For this review, take the finished solid that the model builds, in its own axes (mm). A direction names the side the tool comes from. Round coordinates to 2 decimals unless told otherwise and drop trailing zeros. Order: outer loops, then holes, each group sorted by start corner. A loop starts at its lowest first (then second) coordinate and runs counter-clockwise, first axis right, second up. Notation, with made-up numbers: (30.25, -23.75) -> (54.25, -23.75) arc R27 ccw to (54.25, -3.75) -> close; hole circle Ø7 at (34.5, 21.5). An arc over 180 degrees is marked (long way). Answer in a Markdown table with one row per item.
```python
from build123d import *

# Parameters (mm, degrees)
PAD_DEPTH       = 40
POCKET_DEPTH    = 19
POCKET001_DEPTH = 19
FILLET_R        = 1
FILLET001_R     = 1.8


with BuildPart() as part:
    # Sketch → Pad (new body)
    with BuildSketch(Plane.XY):
        Polygon((0, 0), (0, -55), (5, -55), (45, -15), (45, 0), (41, 0), (41, -10), (5, -10), (5, 0), align=None)
    extrude(amount=PAD_DEPTH)

    # Sketch001 (on Face10 of Pad) → Pocket (cut)
    with BuildSketch(Plane(origin=(0, 0, 0), x_dir=(1, 0, 0), z_dir=(0, 0, -1))):
        Polygon((5, 12.5), (5, 50.5), (41, 12.5), align=None)
    extrude(amount=-POCKET_DEPTH, mode=Mode.SUBTRACT)

    # Sketch002 (on Face5 of Pocket) → Pocket001 (cut)
    with BuildSketch(Plane.XY.offset(40)):
        Polygon((5, -12.5), (41, -12.5), (5, -50.5), align=None)
    extrude(amount=-POCKET001_DEPTH, mode=Mode.SUBTRACT)

    # Fillet
    fillet_edges = [part.edges().sort_by_distance(p)[0] for p in [
        (5, 0, 20),
        (5, -10, 20),
        (45, -15, 20),
        (45, 0, 20),
        (41, 0, 20),
        (5, -55, 20),
        (41, -10, 20),
        (41, -12.5, 30.5),
        (5, -12.5, 30.5),
        (5, -50.5, 30.5),
        (5, -12.5, 9.5),
        (5, -50.5, 9.5),
        (41, -12.5, 9.5),
    ]]
    fillet(fillet_edges, radius=FILLET_R)

    # Fillet001
    fillet001_edges = [part.edges().sort_by_distance(p)[0] for p in [
        (23, -10, 40),
        (23, -10, 0),
    ]]
    fillet(fillet001_edges, radius=FILLET001_R)


solid = part.part
```
Q1. Clearance check with flat-ended pins moving along their axes: pin 1 Ø15 at (x, z) = (30.5, 31) entering from -Y; pin 2 Ø15 at (y, z) = (-34, 34) entering from +X; pin 3 Ø10.5 at (x, y) = (17, -26.5) entering from +Z. State where each tip first meets the part, or that it passes through.
Answer key:
| item | result |
|---|---|
| pin 1 | stops at y = -37 |
| pin 2 | stops at x = 33.5 |
| pin 3 | stops at z = 21 |
Q2. The part is to be moulded in two halves that separate along X. For faces 6 (the face through (41, -5, 20)), 7 (the face through (4, -25, 40)), 8 (the face through (24.89, -34.34, 39.49)), say which applies: +X half, -X half, draft (parallel to the pull), parting line (faces both ways), or undercut.
Answer key:
| item | result |
|---|---|
| face 6 | undercut |
| face 7 | draft |
| face 8 | +X half |
Q3. To check wall thickness, follow probe 1 along X at (y, z) = (-9, 36); probe 2 along Z at (x, y) = (6, -46.5); probe 3 along X at (y, z) = (-18, 18). State the ranges of each line that lie inside material, in increasing order.
Answer key:
| item | result |
|---|---|
| probe 1 | x = 0 to 5, 41 to 45 |
| probe 2 | z = 19 to 21 |
| probe 3 | x = 0 to 5, 35.79 to 42 |
Q4. Tool access review of faces 1 (the face through (5, -5, 20)), 2 (the face through (39.6, -13.12, 9.63)), 3 (the face through (43, 0, 20)), 4 (the face through (22, -12.5, 31)), 5 (the face through (41.541, -5.056, 0.513)): name each direction out of +Z, -Z, +X, -X, +Y, -Y from which nothing blocks a thin tool from reaching the whole face with its end or side.
Answer key:
| item | result |
|---|---|
| face 1 | +Z, -Z, +Y |
| face 2 | -Z |
| face 3 | +Z, -Z, +X, -X, +Y |
| face 4 | +Z |
| face 5 | -Z, +Y |
Q5. Take a section at A-A, the plane z = 17.5. Write out the cut boundary in (x, y), then the cut area to 3 significant figures.
Answer key:
| item | result |
|---|---|
| outline | (0, -55) -> (4.59, -55) arc R1 ccw to (5.29, -54.71) -> (44.71, -15.29) arc R1 ccw to (45, -14.59) -> (45, -1) arc R1 ccw to (44, 0) -> (42, 0) arc R1 ccw to (41, -1) -> (41, -9) arc R1 cw to (40, -10) -> (6, -10) arc R1 cw to (5, -9) -> (5, -1) arc R1 ccw to (4, 0) -> (0, 0) -> close; hole (5, -47.99) arc R1 ccw to (6.73, -48.68) -> (39.4, -14.19) arc R1 ccw to (38.68, -12.5) -> (6, -12.5) arc R1 ccw to (5, -13.5) -> close |
| area | 633 mm^2 |
